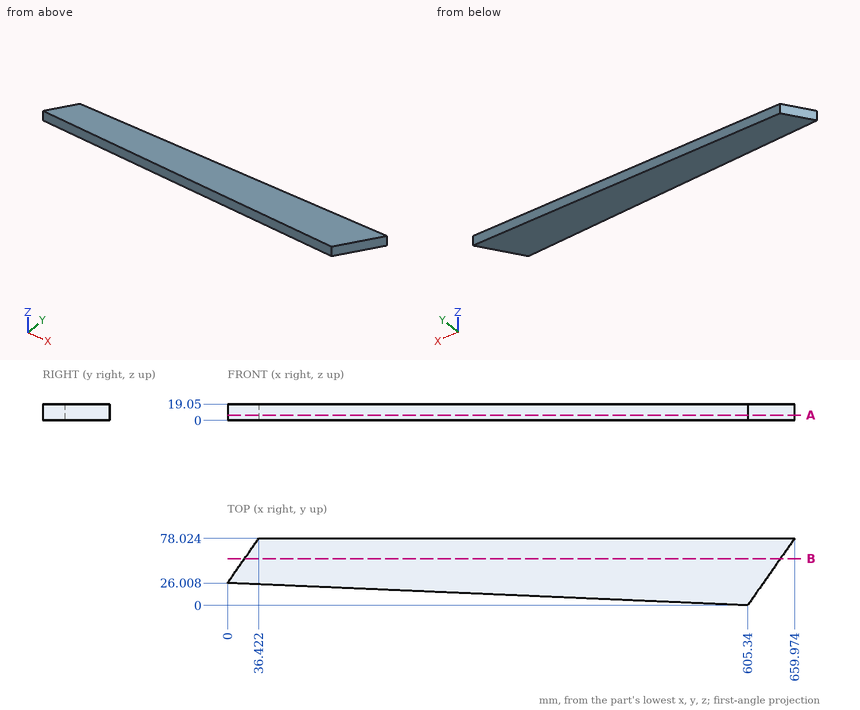
Print and shaded views of the part. All mm, measured from the part's lowest x, y and z. Round coordinates to 2 decimals unless told otherwise and drop trailing zeros. Write each loop counter-clockwise with the first axis right and the second up, starting at its lowest first coordinate (ties: lowest second). Pieces come first, ordered by that corner, then holes. Notation, with made-up numbers: M 45,-1.5 L 99,-1.5 A30 ccw 99,30.5 Z; hole C 63,88 d7. An arc over 180 degrees is marked long. Use a Markdown table: item, result. Add a question column.
1. Slice it at B-B on y = 54.5. Give the cut face in (x, z), then the cut area to 3 significant figures.
2. Slice it at A-A on z = 6. Give the cut face in (x, y) (1 decimal).
3. Flat gauge pins, fed straight in: P1, Ø10, axis at y = 29, z = 15, coming from the +X side; P2, Ø4, axis at x = 249.5, z = 6, coming from the -Y side; P3, Ø6, axis at x = 521.5, z = 3.5, coming from the -Y side. Where does each tip first touch, or does it go through?
4. Drill centre lines: probe 1 along Y at (x, z) = (488, 6) (1 decimal); probe 2 along Y at (x, z) = (548.5, 7.5) (1 decimal); probe 3 along X at (y, z) = (56, 4). Where is each one in solid material? Low to high.
Reply:
| question | item | result |
|---|---|---|
| 1 | outline | M 19.95,0 L 643.5,0 L 643.5,19.05 L 19.95,19.05 Z |
| 1 | area | 11,900 mm^2 |
| 2 | outline | M 0,26 L 605.3,0 L 660,78 L 36.4,78 Z |
| 3 | P1 | stops at x = 629.15 |
| 3 | P2 | stops at y = 15.2 |
| 3 | P3 | stops at y = 3.47 |
| 4 | probe 1 | y = 5 to 78 |
| 4 | probe 2 | y = 2.4 to 78 |
| 4 | probe 3 | x = 21 to 644.55 |
